```python
from build123d import *

# Parameters (mm, degrees)
SKETCH1_W                                           = 120
SKETCH1_H                                           = 90
BOSS_EXTRUDE1_DEPTH                                 = 1.66
CSK_FOR_M3_COUNTERSUNK_FLAT_HEAD_SCREW1_D           = 3.4
CSK_FOR_M3_COUNTERSUNK_FLAT_HEAD_SCREW1_DEPTH       = 30
CSK_FOR_M3_COUNTERSUNK_FLAT_HEAD_SCREW1_CSINK_D     = 6.3
CSK_FOR_M3_COUNTERSUNK_FLAT_HEAD_SCREW1_CSINK_ANGLE = 90
CSK_FOR_M3_COUNTERSUNK_FLAT_HEAD_SCREW1_TIP         = 1.021463052


with BuildPart() as part:
    # Sketch1 → Boss-Extrude1 (new body)
    with BuildSketch(Plane.XY):
        with Locations((60, 45)):
            Rectangle(SKETCH1_W, SKETCH1_H)
    extrude(amount=BOSS_EXTRUDE1_DEPTH)

    # CSK for M3 Countersunk Flat Head Screw1
    with Locations(Plane(origin=(0, 0, 0), x_dir=(-1, 0, 0), z_dir=(0, 0, -1))):
        with Locations((-5, 5), (-5, 85), (-115, 85), (-115, 5)):
            CounterSinkHole(CSK_FOR_M3_COUNTERSUNK_FLAT_HEAD_SCREW1_D / 2, CSK_FOR_M3_COUNTERSUNK_FLAT_HEAD_SCREW1_CSINK_D / 2, depth=CSK_FOR_M3_COUNTERSUNK_FLAT_HEAD_SCREW1_DEPTH, counter_sink_angle=CSK_FOR_M3_COUNTERSUNK_FLAT_HEAD_SCREW1_CSINK_ANGLE)
            with Locations((0, 0, -(CSK_FOR_M3_COUNTERSUNK_FLAT_HEAD_SCREW1_DEPTH + CSK_FOR_M3_COUNTERSUNK_FLAT_HEAD_SCREW1_TIP / 2))):  # 118° drill point
                Cone(0, CSK_FOR_M3_COUNTERSUNK_FLAT_HEAD_SCREW1_D / 2, CSK_FOR_M3_COUNTERSUNK_FLAT_HEAD_SCREW1_TIP, mode=Mode.SUBTRACT)


solid = part.part
```
Geometry check sheet. Reference: the model listing, model coordinates, mm. Give positions to 0.01 mm unless a question says otherwise; leave off trailing zeros. Order: outer loops, then holes, each group sorted by start corner. A loop starts at its lowest first (then second) coordinate and runs counter-clockwise, first axis right, second up.
1. Thickness scan on L1, parallel to Y at x = 115, z = 1.6; L2, parallel to X at y = 85, z = 1.5. Record the ranges inside material, lowest first.
2. Gauge pin test, flat ends, axial feed: pin 1 Ø3 at (x, y) = (115, 85) entering from -Z; pin 2 Ø4.5 at (x, y) = (5, 85) entering from -Z. Record the tip position at first contact, or that the pin passes through.
3. Section check B-B, the plane y = 85. Enter the section's corners in (x, z).
4. Section check A-A, the plane x = 5. Enter the section's corners in (y, z), and give its area (3 significant figures).
Values follow:
1. L1: y = 0 to 3.3, 6.7 to 83.3, 86.7 to 90
1. L2: x = 0 to 3.3, 6.7 to 113.3, 116.7 to 120
2. pin 1: passes through
2. pin 2: stops at z = 0.9
3. outline: (0, 0) - (1.85, 0) - (3.3, 1.45) - (3.3, 1.66) - (0, 1.66) - close; (6.7, 1.45) - (8.15, 0) - (111.85, 0) - (113.3, 1.45) - (113.3, 1.66) - (6.7, 1.66) - close; (116.7, 1.45) - (118.15, 0) - (120, 0) - (120, 1.66) - (116.7, 1.66) - close
4. outline: (0, 0) - (1.85, 0) - (3.3, 1.45) - (3.3, 1.66) - (0, 1.66) - close; (6.7, 1.45) - (8.15, 0) - (81.85, 0) - (83.3, 1.45) - (83.3, 1.66) - (6.7, 1.66) - close; (86.7, 1.45) - (88.15, 0) - (90, 0) - (90, 1.66) - (86.7, 1.66) - close
4. area: 134 mm2
